from build123d import *

# Parameters (mm, degrees)
F1_DEPTH      = 1150
F1_DEPTH_BACK = 1150
F3_DEPTH      = 25
F3_DEPTH_BACK = 25


with BuildPart() as f1:
    # F0 (on Right) → F1 (new body, two sides)
    with BuildSketch(Plane.YZ) as f1_sk:
        with BuildLine():
            ThreePointArc((-20, -28), (-19.4142135624, -29.4142135624), (-18, -30))
            Line((-18, -30), (18, -30))
            ThreePointArc((18, -30), (19.4142135624, -29.4142135624), (20, -28))
            Line((20, -28), (20, 28))
            ThreePointArc((20, 28), (19.4142135624, 29.4142135624), (18, 30))
            Line((18, 30), (-18, 30))
            ThreePointArc((-18, 30), (-19.4142135624, 29.4142135624), (-20, 28))
            Line((-20, 28), (-20, -28))
        make_face()
        with BuildLine():
            Line((17, -28), (-17, -28))
            ThreePointArc((-17, -28), (-17.7071067812, -27.7071067812), (-18, -27))
            Line((-18, -27), (-18, 27))
            ThreePointArc((-18, 27), (-17.7071067812, 27.7071067812), (-17, 28))
            Line((-17, 28), (17, 28))
            ThreePointArc((17, 28), (17.7071067812, 27.7071067812), (18, 27))
            Line((18, 27), (18, -27))
            ThreePointArc((18, -27), (17.7071067812, -27.7071067812), (17, -28))
        make_face(mode=Mode.SUBTRACT)
    extrude(amount=F1_DEPTH)
    extrude(f1_sk.sketch, amount=-F1_DEPTH_BACK)

    # F2 (on Front) → F3 (cut, two sides)
    with BuildSketch(Plane.XZ) as f3_sk:
        Polygon((-1150, 30), (-1150, -30), (-1090, 30), align=None)
        Polygon((1090, 30), (1150, -30), (1150, 30), align=None)
    extrude(amount=-F3_DEPTH, mode=Mode.SUBTRACT)
    extrude(f3_sk.sketch, amount=F3_DEPTH_BACK, mode=Mode.SUBTRACT)


solid = f1.part
Source: CAD feature listing. Evaluate the final solid. Frame: model axes, mm. A direction names the side the tool comes from. Coordinates: 2 decimals unless noted, no trailing zeros. Order: outer loops, then holes, each group sorted by start corner. A loop starts at its lowest first (then second) coordinate and runs counter-clockwise, first axis right, second up. Notation, with made-up numbers: M -3.75,7 L 14.25,7 A26 ccw 14.25,43 Z; hole C 69,21.5 d2. An arc over 180 degrees is marked long. Write each question's results on one line, items separated by ' | '. Start each with the question number.
Item 1: Line query: probe 1 along Z at (x, y) = (639, -1.5); probe 2 along Y at (x, z) = (321, -18.5); probe 3 along X at (y, z) = (18.5, 14.5). Output: solid intervals per line, ascending.
Item 2: Cut plane B-B (x = 548). Return loops of the section in (y, z).
Item 3: Draft query along Z for faces 1 (the face through (15, 0, 30)), 2 (the face through (16, 0, -30)), 3 (the face through (16, -18, 0)). Return one class per face: pulls with the +Z half, pulls with the -Z half, needs draft (parallel to the pull), parting line crosses it, or undercut.
Item 4: Cut plane A-A (z = -12.5). Return loops of the section in (x, y).
Item 5: Set-up query: faces 4 (the face through (16, 18, 0)), 5 (the face through (1118, -19, 2)). Return all of +Z, -Z, +X, -X, +Y, -Y with unobstructed straight access to the full face (end or side cutting, diameter ignored); none if empty.
Item 6: Cut plane C-C (y = -11). Return loops of the section in (x, z), and give its area (3 significant figures).
Item 7: First-contact query: pin 1 Ø10 at (y, z) = (1, 20) entering from +X. Flat tip, straight axial feed; report the tip coordinate or a pass-through.
Checked values:
1) probe 1: z = -30 to -28, 28 to 30 | probe 2: y = -20 to -18, 18 to 20 | probe 3: x = -1105.5 to 1105.5
2) outline: M -20,-28 A2 ccw -18,-30 L 18,-30 A2 ccw 20,-28 L 20,28 A2 ccw 18,30 L -18,30 A2 ccw -20,28 Z; hole M -18,-27 A1 ccw -17,-28 L 17,-28 A1 ccw 18,-27 L 18,27 A1 ccw 17,28 L -17,28 A1 ccw -18,27 Z
3) face 1: pulls with the +Z half | face 2: pulls with the -Z half | face 3: undercut
4) outline: M -1132.5,-20 L 1132.5,-20 L 1132.5,-18 L -1132.5,-18 Z; M -1132.5,18 L 1132.5,18 L 1132.5,20 L -1132.5,20 Z
5) face 4: +X, -X | face 5: +Z, +X, +Y, -Y
6) outline: M -1150,-30 L 1150,-30 L 1148,-28 L -1148,-28 Z; M -1092,28 L 1092,28 L 1090,30 L -1090,30 Z | area: 8,960 mm2
7) pin 1: passes through
